Can you work these out from the model? Positions are in its coordinate system, mm. Face numbers are marked on the shaded views. Coordinates: 2 decimals unless noted, no trailing zeros. Loops run counter-clockwise (first coordinate to the right, second up) from the corner with the lowest first, then second, coordinate; pieces in that order, holes last. Notation, with made-up numbers: M -10.75,11.25 L 44.25,11.25 A22 cw 44.25,47.25 Z; hole C 23.5,26.25 d9. An arc over 180 degrees is marked long. Return JSON: item names as keys, results as strings. Group by question number.
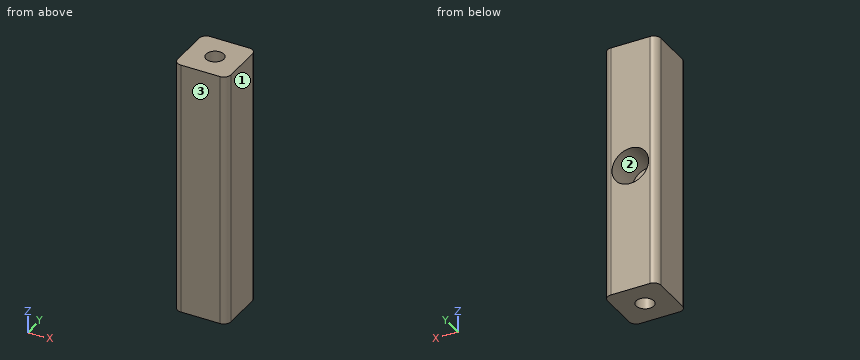
Autodesk Inventor part; units mm, degrees
ref_plane "Work Plane1" through (0, 0, 36) normal (0, 0, 1) x (1, 0, 0)
ref_plane "YZ Plane" through (0, 0, 0) normal (1, 0, 0) x (0, 1, 0)
ref_plane "XZ Plane" through (0, 0, 0) normal (0, 1, 0) x (-1, 0, 0)
sketch "Sketch1" plane through (0, 0, 0) normal (0, 0, 1) x (1, 0, 0)
  line L0 (-7.5, 7.5) -> (7.5, 7.5)
  line L1 (7.5, 7.5) -> (7.5, -7.5)
  line L2 (7.5, -7.5) -> (-7.5, -7.5)
  line L3 (-7.5, -7.5) -> (-7.5, 7.5)
  line L4 (-7.5, 7.5) -> (7.5, -7.5) construction
  line L5 (7.5, 7.5) -> (-7.5, -7.5) construction
  point P0 (0, 0)
  dimension "d0" = 15
  dimension "d1" = 15
extrude "Extrusion1" add sketch "Sketch1" along normal blind 72
sketch "Sketch2" plane through (0, 0, 72) normal (0, 0, 1) x (1, 0, 0)
  circle A0 centre (0, 0) radius 2.5
  dimension "d4" = 5
extrude "Extrusion2" cut sketch "Sketch2" against normal blind 14
ref_plane "Work Plane1" through (0, 0, 36) normal (0, 0, 1) x (1, 0, 0)
mirror "Mirror1" about plane through (0, 0, 36) normal (0, 0, 1) of "Extrusion2"
fillet "Fillet1" radius 2 4 edges at (7.5, 7.5, 36) (-7.5, 7.5, 36) (7.5, -7.5, 36) (-7.5, -7.5, 36)
sketch "Sketch3" plane through (-5.5, 7.5, 0) normal (0, 1, 0) x (1, 0, 0)
  line L0 (-2, -72) -> (-2, 0)
  line L1 (-2, -36) -> (13, -36)
  line L2 (13, 0) -> (13, -72)
  circle A0 centre (5.5, -36) radius 5.15
  point P0 (5.5, 0)
  dimension "d8" = 10.3
extrude "Extrusion3" cut sketch "Sketch3" against normal blind 10
properties part number "FP V2 Claw Connector"
1) For pin 1 (2.5 mm diameter, centred on x = -1, y = -0.5, fed in from -Z); pin 2 (5 mm diameter, centred on x = 1.5, z = 36.5, fed in from +Y), each with a flat end and sliding along its axis, tell me the tip position at first contact or that it passes through.
2) If I drill on line 1 (Y direction, x = 0, z = 3.25); line 2 (X direction, y = -0.25, z = 59); line 3 (Z direction, x = 0, y = 0.5), over which ranges is the centre line in solid material (lowest first)? Write a range as from..to.
3) Suppose I cut it at B-B, the plane z = 50. List the corners of the cut face in (x, y) for me.
4) If we mould it in two halves opening along X, with no side actions, what happens to the marked faces 1, 2 and 3? For each: +X half, -X half, draft (parallel to the pull), parting line (faces both ways), or undercut.
5) Suppose I cut it at C-C, the plane x = 0. List the corners of the cut face in (y, z) for me, then the cut area to 3 significant figures.
6) Suppose I cut it at A-A, the plane y = 0. List the corners of the cut face in (x, z) for me, then the cut area to 3 significant figures.
7) Suppose I cut it at D-D, the plane z = 36. List the corners of the cut face in (x, y) for me, then the cut area to 3 significant figures.
Returned:
{
 "1": {"pin 1": "stops at z = 14", "pin 2": "stops at y = -2.5"},
 "2": {"line 1": "y = -7.5..-2.5, 2.5..7.5", "line 2": "x = -7.5..-2.49, 2.49..7.5", "line 3": "z = 14..30.85, 41.15..58"},
 "3": {"outline": "M -7.5,-5.5 A2 ccw -5.5,-7.5 L 5.5,-7.5 A2 ccw 7.5,-5.5 L 7.5,5.5 A2 ccw 5.5,7.5 L -5.5,7.5 A2 ccw -7.5,5.5 Z"},
 "4": {"face 1": "+X half", "face 2": "undercut", "face 3": "draft"},
 "5": {"outline": "M -7.5,0 L -2.5,0 L -2.5,14 L 2.5,14 L 2.5,0 L 7.5,0 L 7.5,30.85 L -2.5,30.85 L -2.5,41.15 L 7.5,41.15 L 7.5,72 L 2.5,72 L 2.5,58 L -2.5,58 L -2.5,72 L -7.5,72 Z", "area": "837 mm²"},
 "6": {"outline": "M -7.5,0 L -2.5,0 L -2.5,14 L 2.5,14 L 2.5,0 L 7.5,0 L 7.5,72 L 2.5,72 L 2.5,58 L -2.5,58 L -2.5,72 L -7.5,72 Z; hole C 0,36 d10.3", "area": "857 mm²"},
 "7": {"outline": "M -7.5,-5.5 A2 ccw -5.5,-7.5 L 5.5,-7.5 A2 ccw 7.5,-5.5 L 7.5,5.5 A2 ccw 5.5,7.5 L 5.15,7.5 L 5.15,-2.5 L -5.15,-2.5 L -5.15,7.5 L -5.5,7.5 A2 ccw -7.5,5.5 Z", "area": "119 mm²"}
}
